Verification items for the finished model (mm, model axes). A direction names the side the tool comes from. Round coordinates to 2 decimals unless told otherwise and drop trailing zeros. Write each loop counter-clockwise with the first axis right and the second up, starting at its lowest first coordinate (ties: lowest second). Pieces come first, ordered by that corner, then holes. Notation, with made-up numbers: M -4,56 L 7,56 A27 ccw 7,94 Z; hole C 8.5,-34.75 d4. An arc over 180 degrees is marked long. Answer in a Markdown table with one row per item. Add a question column.
1. Sectioned sample at C-C on y = -11. Record the cut outline in (x, z).
2. Draft check along Y on faces 1 (the flat face through (0, -20, 2)), 2 (the flat face through (0, 0, 0)), 3 (the flat face through (21, 13.2, 3)). Enter one of: pulls with the +Y half, pulls with the -Y half, needs draft (parallel to the pull), parting line crosses it, or undercut.
3. Sectioned sample at A-A on x = 21.5. Record the cut outline in (y, z), plus the area to 3 significant figures.
4. Material ranges on probe 1 along Y at (x, z) = (18, 2.5); probe 2 along X at (y, z) = (11, 4.65); probe 3 along Y at (x, z) = (-28, 1.9), recorded low to high.
5. Set-up check for faces 4 (the cylindrical face through (28.28, -10.95, 2.54)), 5 (the flat face through (-35, 0, 2)): record each of +Z, -Z, +X, -X, +Y, -Y from which the full face is reachable in a straight line by a thin tool's end or side.
6. Sectioned sample at B-B on z = 1.5. Record the cut outline in (x, y).
```python
from build123d import *

# Parameters (mm, degrees)
SKETCH1_W            = 70
SKETCH1_H            = 40
BOSS_EXTRUDE1_DEPTH  = 5
CUT_EXTRUDE1_DEPTH   = 41.620192023
MIRROR3_COPY_1_DEPTH = 41.620192023


with BuildPart() as part:
    # Sketch1 → Boss-Extrude1 (new body)
    with BuildSketch(Plane.XY):
        Rectangle(SKETCH1_W, SKETCH1_H)
    extrude(amount=BOSS_EXTRUDE1_DEPTH)

    # Sketch3 → Cut-Extrude1 (cut, through all)
    with BuildSketch(Plane.XY.offset(5)):
        with BuildLine():
            Line((-26.080867749, 13.2), (-15, 13.2))
            ThreePointArc((-15, 13.2), (-12.8, 11), (-15, 8.8))
            Line((-15, 8.8), (-26.080867749, 8.8))
            ThreePointArc((-26.080867749, 8.8), (-28.280867749, 11), (-26.080867749, 13.2))
        make_face()
    cut_extrude1 = extrude(amount=-CUT_EXTRUDE1_DEPTH, mode=Mode.SUBTRACT)

    # Mirror2: Cut-Extrude1 across plane
    add(cut_extrude1.mirror(Plane(origin=(0, 0, 0), x_dir=(0, 0, 1), z_dir=(1, 0, 0))), mode=Mode.SUBTRACT)

    # Mirror3: Cut-Extrude1 across plane
    add(cut_extrude1.mirror(Plane.ZX), mode=Mode.SUBTRACT)

    # Mirror3 copy 1 sketch → Mirror3 copy 1 (cut, through all)
    with BuildSketch(Plane(origin=(0, 0, 5), x_dir=(-1, 0, 0), z_dir=(0, 0, 1))):
        with BuildLine():
            Line((-26.080867749, 13.2), (-15, 13.2))
            ThreePointArc((-15, 13.2), (-12.8, 11), (-15, 8.8))
            Line((-15, 8.8), (-26.080867749, 8.8))
            ThreePointArc((-26.080867749, 8.8), (-28.280867749, 11), (-26.080867749, 13.2))
        make_face()
    extrude(amount=-MIRROR3_COPY_1_DEPTH, mode=Mode.SUBTRACT)


solid = part.part
```
Geometry check:
| question | item | result |
|---|---|---|
| 1 | outline | M -35,0 L -28.28,0 L -28.28,5 L -35,5 Z; M -12.8,0 L 12.8,0 L 12.8,5 L -12.8,5 Z; M 28.28,0 L 35,0 L 35,5 L 28.28,5 Z |
| 2 | face 1 | pulls with the -Y half |
| 2 | face 2 | needs draft |
| 2 | face 3 | undercut |
| 3 | outline | M -20,0 L -13.2,0 L -13.2,5 L -20,5 Z; M -8.8,0 L 8.8,0 L 8.8,5 L -8.8,5 Z; M 13.2,0 L 20,0 L 20,5 L 13.2,5 Z |
| 3 | area | 156 mm2 |
| 4 | probe 1 | y = -20 to -13.2, -8.8 to 8.8, 13.2 to 20 |
| 4 | probe 2 | x = -35 to -28.28, -12.8 to 12.8, 28.28 to 35 |
| 4 | probe 3 | y = -20 to -12.08, -9.92 to 9.92, 12.08 to 20 |
| 5 | face 4 | +Z, -Z |
| 5 | face 5 | +Z, -Z, -X, +Y, -Y |
| 6 | outline | M -35,-20 L 35,-20 L 35,20 L -35,20 Z; hole M -26.08,-13.2 L -15,-13.2 A2.2 ccw -15,-8.8 L -26.08,-8.8 A2.2 ccw Z; hole M -26.08,8.8 L -15,8.8 A2.2 ccw -15,13.2 L -26.08,13.2 A2.2 ccw Z; hole M 15,-13.2 L 26.08,-13.2 A2.2 ccw 26.08,-8.8 L 15,-8.8 A2.2 ccw Z; hole M 15,8.8 L 26.08,8.8 A2.2 ccw 26.08,13.2 L 15,13.2 A2.2 ccw Z |
